Read the model definition and answer for the solid it produces. Units are mm, in the model's axes. Coordinates: 2 decimals unless noted, no trailing zeros.
1) Find the intervals of material crossed by line 1 (Y direction, x = 13.5, z = 0.7), in increasing order.
2) Determine the mould class of faces 1 (the face through (16, 1, 0)), 2 (the face through (19.25, 1.57, 0.49)), 3 (the face through (0, 1.1, 0.5)) for opening direction X: +X half, -X half, draft (parallel to the pull), parting line (faces both ways), or undercut.
3) The part is cut by section A-A (y = 1.3). Give the number of separate pieces and of enclosed holes in the cut face, then the cut area to 3 significant figures.
Autodesk Inventor part; units mm, degrees
ref_plane "YZ Plane" through (0, 0, 0) normal (1, 0, 0) x (0, 1, 0)
ref_plane "XZ Plane" through (0, 0, 0) normal (0, 1, 0) x (-1, 0, 0)
ref_plane "XY Plane" through (0, 0, 0) normal (0, 0, 1) x (1, 0, 0)
sketch "草圖2" plane through (0, 0, 0) normal (0, 0, 1) x (1, 0, 0)
  line L0 (0, 0) -> (32.9867, 0)
  line L1 (32.9867, 0) -> (32.9867, 2.125)
  line L2 (32.9867, 2.125) -> (0, 2.125)
  line L3 (0, 2.125) -> (0, 0)
  line L4 (0, 1) -> (32.9867, 1) construction
  line L5 (0.1974, 2.125) -> (0.6069, 1)
  line L6 (0.9639, 1) -> (1.3734, 2.125)
  line L7 (0.7854, 2.125) -> (0.7854, 1) construction
  line L8 (0, 0.875) -> (32.9867, 0.875) construction
  arc A0 (0.6069, 1) -> (0.9639, 1) centre (0.7854, 1.065) ccw
  line L9 (0, 1.625) -> (32.9867, 1.625) construction
  line L10 (2.5347, 1) -> (2.9442, 2.125)
  arc A1 (2.1777, 1) -> (2.5347, 1) centre (2.3562, 1.065) ccw
  line L11 (1.7682, 2.125) -> (2.1777, 1)
  line L12 (4.1055, 1) -> (4.515, 2.125)
  arc A2 (3.7484, 1) -> (4.1055, 1) centre (3.927, 1.065) ccw
  line L13 (3.339, 2.125) -> (3.7484, 1)
  line L14 (5.6763, 1) -> (6.0858, 2.125)
  arc A3 (5.3192, 1) -> (5.6763, 1) centre (5.4978, 1.065) ccw
  line L15 (4.9098, 2.125) -> (5.3192, 1)
  line L16 (7.2471, 1) -> (7.6566, 2.125)
  arc A4 (6.89, 1) -> (7.2471, 1) centre (7.0686, 1.065) ccw
  line L17 (6.4806, 2.125) -> (6.89, 1)
  line L18 (8.8179, 1) -> (9.2274, 2.125)
  arc A5 (8.4608, 1) -> (8.8179, 1) centre (8.6394, 1.065) ccw
  line L19 (8.0514, 2.125) -> (8.4608, 1)
  line L20 (10.3887, 1) -> (10.7982, 2.125)
  arc A6 (10.0316, 1) -> (10.3887, 1) centre (10.2102, 1.065) ccw
  line L21 (9.6222, 2.125) -> (10.0316, 1)
  line L22 (11.9595, 1) -> (12.369, 2.125)
  arc A7 (11.6024, 1) -> (11.9595, 1) centre (11.781, 1.065) ccw
  line L23 (11.193, 2.125) -> (11.6024, 1)
  line L24 (13.5303, 1) -> (13.9398, 2.125)
  arc A8 (13.1732, 1) -> (13.5303, 1) centre (13.3518, 1.065) ccw
  line L25 (12.7638, 2.125) -> (13.1732, 1)
  line L26 (15.1011, 1) -> (15.5106, 2.125)
  arc A9 (14.744, 1) -> (15.1011, 1) centre (14.9226, 1.065) ccw
  line L27 (14.3346, 2.125) -> (14.744, 1)
  line L28 (16.6719, 1) -> (17.0814, 2.125)
  arc A10 (16.3148, 1) -> (16.6719, 1) centre (16.4934, 1.065) ccw
  line L29 (15.9054, 2.125) -> (16.3148, 1)
  line L30 (18.2427, 1) -> (18.6522, 2.125)
  arc A11 (17.8856, 1) -> (18.2427, 1) centre (18.0642, 1.065) ccw
  line L31 (17.4762, 2.125) -> (17.8856, 1)
  line L32 (19.8135, 1) -> (20.223, 2.125)
  arc A12 (19.4564, 1) -> (19.8135, 1) centre (19.635, 1.065) ccw
  line L33 (19.047, 2.125) -> (19.4564, 1)
  line L34 (21.3843, 1) -> (21.7938, 2.125)
  arc A13 (21.0272, 1) -> (21.3843, 1) centre (21.2058, 1.065) ccw
  line L35 (20.6177, 2.125) -> (21.0272, 1)
  line L36 (22.9551, 1) -> (23.3645, 2.125)
  arc A14 (22.598, 1) -> (22.9551, 1) centre (22.7765, 1.065) ccw
  line L37 (22.1885, 2.125) -> (22.598, 1)
  line L38 (24.5259, 1) -> (24.9353, 2.125)
  arc A15 (24.1688, 1) -> (24.5259, 1) centre (24.3473, 1.065) ccw
  line L39 (23.7593, 2.125) -> (24.1688, 1)
  line L40 (26.0967, 1) -> (26.5061, 2.125)
  arc A16 (25.7396, 1) -> (26.0967, 1) centre (25.9181, 1.065) ccw
  line L41 (25.3301, 2.125) -> (25.7396, 1)
  line L42 (27.6675, 1) -> (28.0769, 2.125)
  arc A17 (27.3104, 1) -> (27.6675, 1) centre (27.4889, 1.065) ccw
  line L43 (26.9009, 2.125) -> (27.3104, 1)
  line L44 (29.2383, 1) -> (29.6477, 2.125)
  arc A18 (28.8812, 1) -> (29.2383, 1) centre (29.0597, 1.065) ccw
  line L45 (28.4717, 2.125) -> (28.8812, 1)
  line L46 (30.8091, 1) -> (31.2185, 2.125)
  arc A19 (30.452, 1) -> (30.8091, 1) centre (30.6305, 1.065) ccw
  line L47 (30.0425, 2.125) -> (30.452, 1)
  line L48 (32.3799, 1) -> (32.7893, 2.125)
  arc A20 (32.0228, 1) -> (32.3799, 1) centre (32.2013, 1.065) ccw
  line L49 (31.6133, 2.125) -> (32.0228, 1)
  point P0 (0.7854, 0.5095)
  point P1 (0.7854, 0.875)
  point P2 (2.3562, 0.5095)
  point P3 (3.927, 0.5095)
  point P4 (5.4978, 0.5095)
  point P5 (7.0686, 0.5095)
  point P6 (8.6394, 0.5095)
  point P7 (10.2102, 0.5095)
  point P8 (11.781, 0.5095)
  point P9 (13.3518, 0.5095)
  point P10 (14.9226, 0.5095)
  point P11 (16.4934, 0.5095)
  point P12 (18.0642, 0.5095)
  point P13 (19.635, 0.5095)
  point P14 (21.2058, 0.5095)
  point P15 (22.7765, 0.5095)
  point P16 (24.3473, 0.5095)
  point P17 (25.9181, 0.5095)
  point P18 (27.4889, 0.5095)
  point P19 (29.0597, 0.5095)
  point P20 (30.6305, 0.5095)
  point P21 (32.2013, 0.5095)
  point P22 (32.7893, 2.125)
  point P23 (31.6133, 2.125)
  point P24 (31.2185, 2.125)
  point P25 (30.0425, 2.125)
  point P26 (29.6477, 2.125)
  point P27 (28.4717, 2.125)
  point P28 (28.0769, 2.125)
  point P29 (26.9009, 2.125)
  point P30 (26.5061, 2.125)
  point P31 (25.3301, 2.125)
  point P32 (24.9353, 2.125)
  point P33 (23.7593, 2.125)
  point P34 (23.3645, 2.125)
  point P35 (22.1885, 2.125)
  point P36 (21.7938, 2.125)
  point P37 (20.6177, 2.125)
  point P38 (20.223, 2.125)
  point P39 (19.047, 2.125)
  point P40 (18.6522, 2.125)
  point P41 (17.4762, 2.125)
  point P42 (17.0814, 2.125)
  point P43 (15.9054, 2.125)
  point P44 (15.5106, 2.125)
  point P45 (14.3346, 2.125)
  point P46 (13.9398, 2.125)
  point P47 (12.7638, 2.125)
  point P48 (12.369, 2.125)
  point P49 (11.193, 2.125)
  point P50 (10.7982, 2.125)
  point P51 (9.6222, 2.125)
  point P52 (9.2274, 2.125)
  point P53 (8.0514, 2.125)
  point P54 (7.6566, 2.125)
  point P55 (6.4806, 2.125)
  point P56 (6.0858, 2.125)
  point P57 (4.9098, 2.125)
  point P58 (4.515, 2.125)
  point P59 (3.339, 2.125)
  point P60 (2.9442, 2.125)
  point P61 (1.7682, 2.125)
  dimension "d17" = 32.9867
  dimension "d18" = 2.125
  dimension "d19" = 1.125
  dimension "d20" = 0.7854
  dimension "d23" = 20
  dimension "d24" = 20
  dimension "d25" = 0.125
  dimension "d26" = 0.19
  dimension "d37" = 0.5
  dimension "d40" = 1.5708
extrude "擠出3" add sketch "草圖2" along normal blind 1 contours L3 L2 L5 A0 L6 L11 A1 L10 L13 A2 L12 L15 A3 L14 L17 A4 L16 L19 A5 L18 L21 A6 L20 L23 A7 L22 L25 A8 L24 L27 A9 L26 L29 A10 L28 L31 A11 L30 L33 A12 L32 L35 A13 L34 L37 A14 L36 L39 A15 L38 L41 A16 L40 L43 A17 L42 L45 A18 L44 L47 A19 L46 L49 A20 L48 L1 L0
equation "\"d17\" = rack_length"
equation "\"d19\" = whole_depth"
equation "\"d20\" = tooth_thickness"
equation "\"d23\" = pressure_angle"
equation "\"d24\" = pressure_angle"
equation "\"d25\" = rack_dedendum"
equation "\"d26\" = fillet_radius"
equation "\"d37\" = addendum"
equation "\"d40\" = circular_pitch"
equation "\"whole_depth\" = 2.25 * module"
equation "\"tooth_thickness\" = 1.5708 * module"
equation "\"circular_pitch\" = 3.14159 * module"
equation "\"addendum\" = module"
equation "\"dedendum\" = 1.25 * module"
equation "\"addendum_diameter\" = pitch_diameter + 2 * addendum"
equation "\"dedendum_diameter\" = pitch_diameter - 2 * dedendum"
equation "\"pressure_angle\" = 20deg"
equation "\"fillet_radius\" = 0.38 * module"
equation "\"rack_dedendum\" = 0.25 * module"
properties part number "齒條"
Reported:
1. line 1: y = 0 to 0.95
2. face 1: draft
2. face 2: undercut
2. face 3: -X half
3. separate pieces: 22
3. enclosed holes: 0
3. area: 20.9 mm2
